```python
from build123d import *

# Parameters (mm, degrees)
SKETCH1_W           = 23
SKETCH1_H           = 12
BOSS_EXTRUDE1_DEPTH = 19.5
SKETCH2_W           = 4.5
SKETCH2_H           = 12
SKETCH2_W_2         = 23
BOSS_EXTRUDE2_DEPTH = 2
SKETCH3_W           = 23
SKETCH3_H           = 12
BOSS_EXTRUDE3_DEPTH = 4
BOSS_EXTRUDE4_DEPTH = 3
SKETCH5_R           = 3
BOSS_EXTRUDE5_DEPTH = 3.5


with BuildPart() as part:
    # Sketch1 → Boss-Extrude1 (new body)
    with BuildSketch(Plane(origin=(0, 0, 0), x_dir=(1, 0, 0), z_dir=(0, 1, 0))):
        with Locations((11.5, 6)):
            Rectangle(SKETCH1_W, SKETCH1_H)
    extrude(amount=BOSS_EXTRUDE1_DEPTH)

    # Sketch2 → Boss-Extrude2 (add)
    with BuildSketch(Plane(origin=(0, 19.5, 0), x_dir=(1, 0, 0), z_dir=(0, 1, 0))):
        with Locations((-2.25, 6)):
            Rectangle(SKETCH2_W, SKETCH2_H)
        with Locations((25.25, 6)):
            Rectangle(SKETCH2_W, SKETCH2_H)
        with Locations((11.5, 6)):
            Rectangle(SKETCH2_W_2, SKETCH2_H)
    extrude(amount=BOSS_EXTRUDE2_DEPTH)

    # Sketch3 → Boss-Extrude3 (add)
    with BuildSketch(Plane(origin=(0, 21.5, 0), x_dir=(1, 0, 0), z_dir=(0, 1, 0))):
        with Locations((11.5, 6)):
            Rectangle(SKETCH3_W, SKETCH3_H)
    extrude(amount=BOSS_EXTRUDE3_DEPTH)

    # Sketch4 → Boss-Extrude4 (add)
    with BuildSketch(Plane(origin=(0, 25.5, 0), x_dir=(1, 0, 0), z_dir=(0, 1, 0))):
        with BuildLine():
            ThreePointArc((12.757359313, 1.757359313), (14.703899406, 0.456722805), (17, 0))
            ThreePointArc((17, 0), (21.242640687, 1.757359313), (23, 6))
            ThreePointArc((23, 6), (22.543277195, 8.296100594), (21.242640687, 10.242640687))
            Line((21.242640687, 10.242640687), (12.757359313, 1.757359313))
        make_face()
        with BuildLine():
            ThreePointArc((11, 6), (11.456722805, 3.703899406), (12.757359313, 1.757359313))
            Line((12.757359313, 1.757359313), (21.242640687, 10.242640687))
            ThreePointArc((21.242640687, 10.242640687), (19.296100594, 11.543277195), (17, 12))
            ThreePointArc((17, 12), (12.757359313, 10.242640687), (11, 6))
        make_face()
    extrude(amount=BOSS_EXTRUDE4_DEPTH)

    # Sketch5 → Boss-Extrude5 (add)
    with BuildSketch(Plane(origin=(0, 28.5, 0), x_dir=(1, 0, 0), z_dir=(0, 1, 0))):
        with Locations((17, 6)):
            Circle(SKETCH5_R)
    extrude(amount=BOSS_EXTRUDE5_DEPTH)


solid = part.part
```
Model file for the job. Use its own axes, mm. A direction names the side the tool comes from. Coordinates: 2 decimals unless noted, no trailing zeros. Loops run counter-clockwise (first coordinate to the right, second up) from the corner with the lowest first, then second, coordinate; pieces in that order, holes last. Notation, with made-up numbers: (75.25, -20) - (98.25, -20) arc R27 cw to (98.25, 12) - close; hole circle Ø8 at (89.25, -1.75). An arc over 180 degrees is marked (long way). Answer as a JSON object with one key per item and string values. Group by question number.
(1) Cut at D-D (x = 19). Give the cut face in (y, z).
(2) Probe line 1 along X through (y, z) = (16.5, -10.75); line 2 along Y through (x, z) = (17, -1.75); line 3 along Y through (x, z) = (1, -11). List the from-to ranges inside material, lowest first.
(3) Tool access for faces 1 (the face through (22, 25.5, -1)), 2 (the face through (25, 19.5, -6)), 3 (the face through (0, 23, -6)), 4 (the face through (0, 10, -6)): list every direction of +Z, -Z, +X, -X, +Y, -Y with a clear straight run to the whole face (end or side of a thin tool).
(4) Cut at A-A (z = -4). Give the cut face in (x, y), then the cut area to 3 significant figures.
(5) Cut at C-C (y = 14). Give the cut face in (x, z), then the cut area to 3 significant figures.
(6) Flat gauge pins, fed straight in: pin 1 (4 mm diameter, centred on y = 13, z = -8, fed in from +X); pin 2 (3.5 mm diameter, centred on x = 26, z = -6.5, fed in from -Y); pin 3 (6 mm diameter, centred on x = 6, z = -6.5, fed in from +Y). Where does each tip first touch, or does it go through?
(7) Cut at B-B (x = 13.5). Give the cut face in (y, z).
Geometry says:
{
 "1": {"outline": "(0, -12) - (25.5, -12) - (25.5, -11.66) - (28.5, -11.66) - (28.5, -8.24) - (32, -8.24) - (32, -3.76) - (28.5, -3.76) - (28.5, -0.34) - (25.5, -0.34) - (25.5, 0) - (0, 0) - close"},
 "2": {"line 1": "x = 0 to 23", "line 2": "y = 0 to 28.5", "line 3": "y = 0 to 25.5"},
 "3": {"face 1": "+Z, +X, +Y", "face 2": "+Z, -Z, +X, -Y", "face 3": "+Z, -Z, -X, +Y", "face 4": "+Z, -Z, -X, -Y"},
 "4": {"outline": "(-4.5, 19.5) - (0, 19.5) - (0, 0) - (23, 0) - (23, 19.5) - (27.5, 19.5) - (27.5, 21.5) - (23, 21.5) - (23, 25.5) - (22.66, 25.5) - (22.66, 28.5) - (19.24, 28.5) - (19.24, 32) - (14.76, 32) - (14.76, 28.5) - (11.34, 28.5) - (11.34, 25.5) - (0, 25.5) - (0, 21.5) - (-4.5, 21.5) - close", "area": "654 mm^2"},
 "5": {"outline": "(0, -12) - (23, -12) - (23, 0) - (0, 0) - close", "area": "276 mm^2"},
 "6": {"pin 1": "stops at x = 23", "pin 2": "stops at y = 19.5", "pin 3": "stops at y = 25.5"},
 "7": {"outline": "(0, -12) - (25.5, -12) - (25.5, -10.87) - (28.5, -10.87) - (28.5, -1.13) - (25.5, -1.13) - (25.5, 0) - (0, 0) - close"}
}
